from build123d import *
from build123d.topology import SkipClean

# Parameters (mm, degrees)
IZIM1_R                       = 67.5
Y_KSEKLIK_EKSTR_ZYON3_DEPTH   = 10
IZIM1_R_2                     = 83.5
Y_KSEKLIK_EKSTR_ZYON3_2_DEPTH = 10
Y_KSEKLIK_EKSTR_ZYON6_DEPTH   = 30
Y_KSEKLIK_EKSTR_ZYON7_START   = 30
IZIM2_4_W                     = 34.219038219
IZIM2_4_H                     = 20
Y_KSEKLIK_EKSTR_ZYON7_DEPTH   = 10
IZIM3_R                       = 1.5
KES_EKSTR_ZYON1_DEPTH         = 20


with BuildPart() as part:
    # izim1 → Y_kseklik-Ekstr_zyon3 (new body)
    with BuildSketch(Plane(origin=(0, 0, 0), x_dir=(1, 0, 0), z_dir=(0, 1, 0))):
        with Locations(Location((0, 0, 0), (0, 0, 270))):
            Circle(IZIM1_R)
        with BuildLine():
            ThreePointArc((22.69357348, 59.306422272), (-31.75, 54.99261314), (-62.707655035, 10))
            Line((-62.707655035, 10), (-57.707655035, 10))
            Line((-57.707655035, 10), (-57.707655035, -10))
            Line((-57.707655035, -10), (-62.707655035, -10))
            ThreePointArc((-62.707655035, -10), (-31.75, -54.99261314), (22.69357348, -59.306422272))
            Line((22.69357348, -59.306422272), (20.19357348, -54.976295253))
            Line((20.19357348, -54.976295253), (37.514081555, -44.976295253))
            Line((37.514081555, -44.976295253), (40.014081555, -49.306422272))
            ThreePointArc((40.014081555, -49.306422272), (63.5, 0), (40.014081555, 49.306422272))
            Line((40.014081555, 49.306422272), (37.514081555, 44.976295253))
            Line((37.514081555, 44.976295253), (20.19357348, 54.976295253))
            Line((20.19357348, 54.976295253), (22.69357348, 59.306422272))
        make_face(mode=Mode.SUBTRACT)
    extrude(amount=Y_KSEKLIK_EKSTR_ZYON3_DEPTH)



with BuildPart() as body_2:
    # izim1 → Y_kseklik-Ekstr_zyon3 2 (new body)
    with BuildSketch(Plane(origin=(0, 0, 0), x_dir=(1, 0, 0), z_dir=(0, 1, 0))):
        with BuildLine():
            Line((54.623600665, -74.610851643), (52.123600665, -70.280724625))
            ThreePointArc((52.123600665, -70.280724625), (87.5, 0), (52.123600665, 70.280724625))
            Line((52.123600665, 70.280724625), (54.623600665, 74.610851643))
            Line((54.623600665, 74.610851643), (37.303092589, 84.610851643))
            Line((37.303092589, 84.610851643), (34.803092589, 80.280724625))
            ThreePointArc((34.803092589, 80.280724625), (-43.75, 75.777222831), (-86.926693254, 10))
            Line((-86.926693254, 10), (-91.926693254, 10))
            Line((-91.926693254, 10), (-91.926693254, -10))
            Line((-91.926693254, -10), (-86.926693254, -10))
            ThreePointArc((-86.926693254, -10), (-43.75, -75.777222831), (34.803092589, -80.280724625))
            Line((34.803092589, -80.280724625), (37.303092589, -84.610851643))
            Line((37.303092589, -84.610851643), (54.623600665, -74.610851643))
        make_face()
        with Locations(Location((0, 0, 0), (0, 0, 270))):
            Circle(IZIM1_R_2, mode=Mode.SUBTRACT)
    extrude(amount=Y_KSEKLIK_EKSTR_ZYON3_2_DEPTH)


with BuildPart() as part_1:
    add(part.part)

    add(body_2.part)  # Y_kseklik-Ekstr_zyon6 merges body 2
    # izim2 → Y_kseklik-Ekstr_zyon6 (add)
    with BuildSketch(Plane(origin=(0, 10, 0), x_dir=(1, 0, 0), z_dir=(0, 1, 0))):
        with BuildLine():
            Line((-57.707655035, -10), (-57.707655035, 10))
            Line((-57.707655035, 10), (-66.755149614, 10))
            ThreePointArc((-66.755149614, 10), (-67.5, 0), (-66.755149614, -10))
            Line((-66.755149614, -10), (-57.707655035, -10))
        make_face()
        with BuildLine():
            ThreePointArc((-82.899034976, -10), (-83.5, 0), (-82.899034976, 10))
            Line((-82.899034976, 10), (-91.926693254, 10))
            Line((-91.926693254, 10), (-91.926693254, -10))
            Line((-91.926693254, -10), (-82.899034976, -10))
        make_face()
        with BuildLine():
            ThreePointArc((42.037828845, 52.811655399), (33.75, 58.456714755), (24.717320769, 62.811655399))
            Line((24.717320769, 62.811655399), (20.19357348, 54.976295253))
            Line((20.19357348, 54.976295253), (37.514081555, 44.976295253))
            Line((37.514081555, 44.976295253), (42.037828845, 52.811655399))
        make_face()
        with BuildLine():
            Line((20.19357348, -54.976295253), (24.717320769, -62.811655399))
            ThreePointArc((24.717320769, -62.811655399), (33.75, -58.456714755), (42.037828845, -52.811655399))
            Line((42.037828845, -52.811655399), (37.514081555, -44.976295253))
            Line((37.514081555, -44.976295253), (20.19357348, -54.976295253))
        make_face()
        with BuildLine():
            Line((37.303092589, 84.610851643), (32.78926345, 76.792670239))
            ThreePointArc((32.78926345, 76.792670239), (41.75, 72.313121216), (50.109771526, 66.792670239))
            Line((50.109771526, 66.792670239), (54.623600665, 74.610851643))
            Line((54.623600665, 74.610851643), (37.303092589, 84.610851643))
        make_face()
        with BuildLine():
            ThreePointArc((50.109771526, -66.792670239), (41.75, -72.313121216), (32.78926345, -76.792670239))
            Line((32.78926345, -76.792670239), (37.303092589, -84.610851643))
            Line((37.303092589, -84.610851643), (54.623600665, -74.610851643))
            Line((54.623600665, -74.610851643), (50.109771526, -66.792670239))
        make_face()
    extrude(amount=Y_KSEKLIK_EKSTR_ZYON6_DEPTH)

    # izim2_4 → Y_kseklik-Ekstr_zyon7 (add)
    with SkipClean():  # the faces are left unmerged after this step: merging them gives an invalid solid
        with BuildSketch(Plane(origin=(0, 10, 0), x_dir=(1, 0, 0), z_dir=(0, 1, 0)).offset(Y_KSEKLIK_EKSTR_ZYON7_START)):
            with Locations((-74.817174145, 0)):
                Rectangle(IZIM2_4_W, IZIM2_4_H)
            Polygon((20.19357348, 54.976295253), (37.514081555, 44.976295253), (54.623600665, 74.610851643), (37.303092589, 84.610851643), align=None)
            Polygon((37.514081555, -44.976295253), (20.19357348, -54.976295253), (37.303092589, -84.610851643), (54.623600665, -74.610851643), align=None)
        extrude(amount=Y_KSEKLIK_EKSTR_ZYON7_DEPTH)

    # izim3 → Kes-Ekstr_zyon1 (cut)
    with SkipClean():  # the faces are left unmerged after this step: merging them gives an invalid solid
        with BuildSketch(Plane(origin=(0, 50, 0), x_dir=(1, 0, 0), z_dir=(0, 1, 0))):
            with Locations(Location((-74.707655035, 0, 0), (0, 0, 270))):
                Circle(IZIM3_R)
            with Locations(Location((37.353827518, 64.698727118, 0), (0, 0, 270))):
                Circle(IZIM3_R)
            with Locations(Location((37.353827518, -64.698727118, 0), (0, 0, 270))):
                Circle(IZIM3_R)
        extrude(amount=-KES_EKSTR_ZYON1_DEPTH, mode=Mode.SUBTRACT)


solid = part_1.part
Can you work these out from the model? Positions are in its coordinate system, mm. A direction names the side the tool comes from. Give positions to 0.01 mm unless a question says otherwise; leave off trailing zeros. Loops run counter-clockwise (first coordinate to the right, second up) from the corner with the lowest first, then second, coordinate; pieces in that order, holes last. Notation, with made-up numbers: M -15,12.25 L 21,12.25 A23 cw 21,21.25 Z; hole C 54.25,-20 d11. An arc over 180 degrees is marked long. One line per item, written item: value. Start each with the question number.
1) If I drill on line 1 (X direction, y = 47.5, z = 0); line 2 (Z direction, x = 37.5, y = 9); line 3 (Y direction, x = -78.5, z = -0.5), over which ranges is the centre line in solid material (lowest first)? Write a range as [from, to].
2) On a 3-axis mill with a long thin cutter (end or side, diameter ignored), from which of +Z, -Z, +X, -X, +Y, -Y can I reach the whole of each face in a straight line? I mean faces 1 (the face through (-31, 10, 56)), 2 (the face through (-57.708, 25, 0)), 3 (the face through (64, 10, 0)), 4 (the face through (-40, 10, -75)). Say none if no direction works.
3) If we section it at D-D, the plane z = 37: Write out the boundary of the cut face in (x, y), and give its area (3 significant figures).
4) If we section it at A-A, the plane y = 5.5: Write out the boundary of the cut face in (x, z).
5) If we section it at C-C, the plane x = 0: Write out the boundary of the cut face in (y, z).
6) I'm going to push flat-ended pins straight in: pin 1 (8 mm diameter, centred on y = 44, z = -60.5, fed in from -X); pin 2 (1 mm diameter, centred on y = 20, z = 11, fed in from +X); pin 3 (7 mm diameter, centred on x = 36.5, z = 70.5, fed in from -Y); pin 4 (10 mm diameter, centred on y = 40, z = -62.5, fed in from +X). Where does each tip first touch, or does it pass through?
7) Thinking about a two-plate mould opening in Z: for faces 5 (the face through (37, 40, 67)), 6 (the face through (-44.736, 4.93, 75.2)), 7 (the face through (-31, 10, -56)), which applies, +Z half, -Z half, draft (parallel to the pull), parting line (faces both ways), or undercut?
8) If we section it at B-B, the plane y = 24.5: Write out the boundary of the cut face in (x, z), and give its area (3 significant figures).
Completed:
1. line 1: x = [-91.93, -76.21], [-73.21, -57.71]
1. line 2: z = [-84.5, -74.61], [-56.12, -44.98], [44.98, 56.12], [74.61, 84.5]
1. line 3: y = [40, 50]
2. face 1: +Z, -X, +Y
2. face 2: +Y, -Y
2. face 3: +X, +Y
2. face 4: -Z, -X, +Y
3. outline: M -79.29,0 L -74.85,0 L -74.85,10 L -79.29,10 Z; M -56.46,0 L -51.61,0 L -51.61,10 L -56.46,10 Z; M 51.61,0 L 56.46,0 L 56.46,10 L 51.61,10 Z; M 74.85,0 L 79.29,0 L 79.29,10 L 74.85,10 Z
3. area: 186 mm^2
4. outline: M -91.93,-10 L -86.93,-10 A87.5 ccw 34.8,-80.28 L 37.3,-84.61 L 54.62,-74.61 L 52.12,-70.28 A87.5 ccw 52.12,70.28 L 54.62,74.61 L 37.3,84.61 L 34.8,80.28 A87.5 ccw -86.93,10 L -91.93,10 Z; C 0,0 d135; hole C 0,0 d167; hole M -62.71,-10 A63.5 ccw 22.69,-59.31 L 20.19,-54.98 L 37.51,-44.98 L 40.01,-49.31 A63.5 ccw 40.01,49.31 L 37.51,44.98 L 20.19,54.98 L 22.69,59.31 A63.5 ccw -62.71,10 L -57.71,10 L -57.71,-10 Z
5. outline: M 0,-87.5 L 10,-87.5 L 10,-83.5 L 0,-83.5 Z; M 0,-67.5 L 10,-67.5 L 10,-63.5 L 0,-63.5 Z; M 0,63.5 L 10,63.5 L 10,67.5 L 0,67.5 Z; M 0,83.5 L 10,83.5 L 10,87.5 L 0,87.5 Z
6. pin 1: stops at x = 21.07
6. pin 2: passes through
6. pin 3: stops at y = 40
6. pin 4: stops at x = 50.52
7. face 5: undercut
7. face 6: +Z half
7. face 7: draft
8. outline: M -91.93,-10 L -82.9,-10 A83.5 cw -82.9,10 L -91.93,10 Z; M -66.76,-10 L -57.71,-10 L -57.71,10 L -66.76,10 A67.5 ccw Z; M 20.19,-54.98 L 24.72,-62.81 A67.5 ccw 42.04,-52.81 L 37.51,-44.98 Z; M 20.19,54.98 L 37.51,44.98 L 42.04,52.81 A67.5 ccw 24.72,62.81 Z; M 32.79,-76.79 L 37.3,-84.61 L 54.62,-74.61 L 50.11,-66.79 A83.5 cw Z; M 32.79,76.79 A83.5 cw 50.11,66.79 L 54.62,74.61 L 37.3,84.61 Z
8. area: 1,090 mm^2
